Read the model definition and answer for the solid it produces. Units are mm, in the model's axes. A direction names the side the tool comes from. Coordinates: 2 decimals unless noted, no trailing zeros. Write each loop counter-clockwise with the first axis right and the second up, starting at its lowest first coordinate (ties: lowest second). Pieces come first, ordered by that corner, then holes. Notation, with made-up numbers: M 71,20.5 L 110,20.5 A23 ccw 110,51.5 Z; hole C 57.25,37.25 d3. An arc over 180 degrees is marked long. Use a Markdown table: item, result. Add a question column.
from build123d import *

# Parameters (mm, degrees)
EXTRUDE_1_DEPTH                           = 1
SKETCH_2_W                                = 1
SKETCH_2_H                                = 10
EXTRUDE_2_DEPTH                           = 1.6
EXTRUDE_3_DEPTH                           = 2
EXTRUDE_4_DEPTH                           = 1
MIRROR_1_AT_THE_SECOND_PLANE_COPY_1_DEPTH = 2
SKETCH_5_R                                = 4.25
CUT_EXTRUDE_1_DEPTH                       = 24.850366873


with BuildPart() as part:
    # 草图1 → 凸台-拉伸1 (new body)
    with BuildSketch(Plane(origin=(0, 0, 0), x_dir=(1, 0, 0), z_dir=(0, 1, 0))):
        with BuildLine():
            Line((2, 0), (9.8, 0))
            ThreePointArc((9.8, 0), (11.214213562, 0.585786438), (11.8, 2))
            Line((11.8, 2), (11.8, 16.8))
            ThreePointArc((11.8, 16.8), (11.214213562, 18.214213562), (9.8, 18.8))
            Line((9.8, 18.8), (2, 18.8))
            ThreePointArc((2, 18.8), (0.585786438, 18.214213562), (0, 16.8))
            Line((0, 16.8), (0, 2))
            ThreePointArc((0, 2), (0.585786438, 0.585786438), (2, 0))
        make_face()
    extrude(amount=EXTRUDE_1_DEPTH)

    # 草图2 → 凸台-拉伸2 (add)
    with BuildSketch(Plane(origin=(0, 1, 0), x_dir=(1, 0, 0), z_dir=(0, 1, 0))):
        with Locations((0.5, 9.4)):
            Rectangle(SKETCH_2_W, SKETCH_2_H)
        with Locations((11.3, 9.4)):
            Rectangle(SKETCH_2_W, SKETCH_2_H)
    extrude(amount=EXTRUDE_2_DEPTH)

    # 草图3 → 凸台-拉伸3 (add, symmetric)
    with BuildSketch(Plane.XY.offset(-9.4)):
        Polygon((0, 2.6), (0, 1.1), (-0.5, 1.1), (-0.5, 2.1), align=None)
    extrude_3 = extrude(amount=EXTRUDE_3_DEPTH, both=True)

    # 草图4 → 凸台-拉伸4 (add)
    with BuildSketch(Plane.XZ):
        with BuildLine():
            Line((2, -19.8), (9.8, -19.8))
            ThreePointArc((9.8, -19.8), (11.921320344, -18.921320344), (12.8, -16.8))
            Line((12.8, -16.8), (12.8, -2))
            ThreePointArc((12.8, -2), (11.921320344, 0.121320344), (9.8, 1))
            Line((9.8, 1), (2, 1))
            ThreePointArc((2, 1), (-0.121320344, 0.121320344), (-1, -2))
            Line((-1, -2), (-1, -16.8))
            ThreePointArc((-1, -16.8), (-0.121320344, -18.921320344), (2, -19.8))
        make_face()
    extrude(amount=EXTRUDE_4_DEPTH)

    # 镜向1: 凸台-拉伸3 across plane
    add(extrude_3.mirror(Plane.XY.offset(-9.4)))

    # 镜向1 at the second plane: 凸台-拉伸3 across plane
    add(extrude_3.mirror(Plane.ZY.offset(-5.9)))

    # 镜向1 at the second plane copy 1 sket → 镜向1 at the second plane copy 1 (add, symmetric)
    with BuildSketch(Plane(origin=(11.8, 0, -9.4), x_dir=(-1, 0, 0), z_dir=(0, 0, -1))):
        Polygon((0, 2.6), (0, 1.1), (-0.5, 1.1), (-0.5, 2.1), align=None)
    extrude(amount=MIRROR_1_AT_THE_SECOND_PLANE_COPY_1_DEPTH, both=True)

    # 草图5 → 切除-拉伸1 (cut, through all)
    with BuildSketch(Plane.XZ.offset(1)):
        with Locations(Location((5.9, -4.5, 0), (0, 0, 270))):
            Circle(SKETCH_5_R)
        with Locations(Location((5.9, -14.3, 0), (0, 0, 270))):
            Circle(SKETCH_5_R)
    extrude(amount=-CUT_EXTRUDE_1_DEPTH, mode=Mode.SUBTRACT)


solid = part.part
Item 1: Find section C-C on x = 4. Give the vertices of the cut face in (y, z).
Item 2: Find section B-B on z = -2.75. Give the vertices of the cut face in (x, y).
Item 3: Determine the mould class of faces 1 (the flat face through (10.8, 2, -9)), 2 (the flat face through (5.8, -0.5, -19.8)), 3 (the flat face through (12.3, 1.6, -9.4)) for opening direction X: pulls with the +X half, pulls with the -X half, needs draft (parallel to the pull), parting line crosses it, or undercut.
Item 4: Find section A-A on x = 5.9. Give the vertices of the cut face in (y, z), then the cut area to 3 significant figures.
Item 5: For faces 4 (the flat face through (11, 2, -4.4)), 5 (the cylindrical face through (0.6, 0.49, -18.23)), 6 (the flat face through (0.5, 1.8, -14.4)), determine the directions among +Z, -Z, +X, -X, +Y, -Y from which every point of the face is accessible in a straight line to the end or side of a thin tool.
Item 6: Consider probe 1 along X at (y, z) = (-0.5, -14.25); probe 2 along X at (y, z) = (2.1, -13.25); probe 3 along Z at (x, y) = (8.25, 0.35). Determine where each line is inside the solid, lowest interval first.
Item 7: Find section D-D on z = -18. Give the vertices of the cut face in (x, y), then the cut area to 3 significant figures.
Item 8: Each of these flat-tipped pins is pushed along its axis until it touches: pin 1 (8 mm diameter, centred on x = 2.5, z = -13.5, fed in from -Y); pin 2 (0.5 mm diameter, centred on y = 1.5, z = -8, fed in from -X); pin 3 (0.8 mm diameter, centred on y = 1.5, z = -10.5, fed in from +X); pin 4 (2 mm diameter, centred on x = 4.5, z = -2, fed in from -Y). Where does it stop, or does it pass through?
Geometry says:
| question | item | result |
|---|---|---|
| 1 | outline | M -1,-19.8 L 0,-19.8 L 0,-18.8 L 1,-18.8 L 1,-18.1 L -1,-18.1 Z; M -1,-10.5 L 1,-10.5 L 1,-8.3 L -1,-8.3 Z; M -1,-0.7 L 1,-0.7 L 1,0 L 0,0 L 0,1 L -1,1 Z |
| 2 | outline | M -1,-1 L 2.03,-1 L 2.03,1 L 0,1 L 0,0 L -1,0 Z; M 9.77,-1 L 12.8,-1 L 12.8,0 L 11.8,0 L 11.8,1 L 9.77,1 Z |
| 3 | face 1 | undercut |
| 3 | face 2 | needs draft |
| 3 | face 3 | pulls with the +X half |
| 4 | outline | M -1,-19.8 L 0,-19.8 L 0,-18.8 L 1,-18.8 L 1,-18.55 L -1,-18.55 Z; M -1,-10.05 L 1,-10.05 L 1,-8.75 L -1,-8.75 Z; M -1,-0.25 L 1,-0.25 L 1,0 L 0,0 L 0,1 L -1,1 Z |
| 4 | area | 5.60 mm2 |
| 5 | face 4 | +Z, +X, -X, +Y |
| 5 | face 5 | -Z, -X, +Y |
| 5 | face 6 | -Z, +X, -X, +Y |
| 6 | probe 1 | x = -1 to 1.65, 10.15 to 12.8 |
| 6 | probe 2 | x = 0 to 1, 10.8 to 11.8 |
| 6 | probe 3 | z = -18.8 to -17.84, -10.76 to -8.04, -0.96 to 0 |
| 7 | outline | M -0.75,-1 L 3.81,-1 L 3.81,1 L 0.4,1 L 0.4,0 L -0.75,0 Z; M 7.99,-1 L 12.55,-1 L 12.55,0 L 11.4,0 L 11.4,1 L 7.99,1 Z |
| 7 | area | 15.9 mm2 |
| 8 | pin 1 | stops at y = -1 |
| 8 | pin 2 | stops at x = -0.5 |
| 8 | pin 3 | stops at x = 12.3 |
| 8 | pin 4 | passes through |
